Part model, mm, in its own coordinate system. Face numbers are marked on the shaded views. A direction names the side the tool comes from. Give positions to 0.01 mm unless a question says otherwise; leave off trailing zeros. Loops run counter-clockwise (first coordinate to the right, second up) from the corner with the lowest first, then second, coordinate; pieces in that order, holes last. Notation, with made-up numbers: M 65,61 L 97,61 A17 ccw 97,87 Z; hole C 14.25,-11.75 d9. An arc over 180 degrees is marked long. Answer in a Markdown table with one row per item.
from build123d import *

# Parameters (mm, degrees)
F1_DEPTH     = 21.2
F2_W         = 14.7
F2_H         = 3.2
F3_DEPTH     = 6.7
F4_R         = 2.6
F5_DEPTH     = 10
F6_W         = 18
F6_H         = 15
F7_DEPTH     = 11.9
F9_DEPTH     = 7.6
F10_T1_DEPTH = 34.5
F10_T3_DEPTH = 27
F11_W        = 14.7
F11_H        = 1.8
F12_DEPTH    = 3.5


# Not quite as in the source:
# - a fillet or chamfer that OpenCascade refuses, or shapes differently, is made with other operations: its cross-section is extruded or revolved along the edge and cut away or added


with BuildPart() as f1:
    # F0 (on Front) → F1 (new body)
    with BuildSketch(Plane.XZ):
        with BuildLine():
            Line((-7.35, 0.194197055), (-7.35, -7.15))
            Line((-7.35, -7.15), (7.35, -7.15))
            Line((7.35, -7.15), (7.35, 0.194197055))
            Line((7.35, 0.194197055), (6.2603328375, 2.1552506672))
            ThreePointArc((6.2603328375, 2.1552506672), (3.3980247264, -0.3840505852), (0, 1.375007837))
            ThreePointArc((0, 1.375007837), (-3.3980247264, -0.3840505852), (-6.2603328375, 2.1552506672))
            Line((-6.2603328375, 2.1552506672), (-7.35, 0.194197055))
        make_face()
        with BuildLine():
            ThreePointArc((0, 4.564992163), (-4.1941925187, 6.1243837001), (-6.2603328375, 2.1552506672))
            ThreePointArc((-6.2603328375, 2.1552506672), (-3.3980247264, -0.3840505852), (0, 1.375007837))
            ThreePointArc((0, 1.375007837), (3.3980247264, -0.3840505852), (6.2603328375, 2.1552506672))
            ThreePointArc((6.2603328375, 2.1552506672), (4.1941925187, 6.1243837001), (0, 4.564992163))
        make_face()
    extrude(amount=F1_DEPTH)

    # F2 (on face) → F3 (cut)
    with BuildSketch(Plane(origin=(0, 0, -7.15), x_dir=(1, 0, 0), z_dir=(0, 0, -1))):
        with Locations((0, 19.6)):
            Rectangle(F2_W, F2_H)
    extrude(amount=-F3_DEPTH, mode=Mode.SUBTRACT)

    # F4 (on face) → F5 (cut)
    with BuildSketch(Plane.XZ.offset(21.2)):
        with Locations((-2.98, 2.97)):
            Circle(F4_R)
        with Locations((2.98, 2.97)):
            Circle(F4_R)
    extrude(amount=-F5_DEPTH, mode=Mode.SUBTRACT)

    # F6 (on face) → F7 (join)
    with BuildSketch(Plane(origin=(0, 0, 0), x_dir=(-1, 0, 0), z_dir=(0, 1, 0))):
        with Locations((0, 3.95)):
            Rectangle(F6_W, F6_H)
    extrude(amount=F7_DEPTH)

    # F8 (on face) → F9 (join)
    with BuildSketch(Plane(origin=(0, 11.9, 0), x_dir=(-1, 0, 0), z_dir=(0, 1, 0))):
        Polygon((-9, -0.05), (-9, -3.55), (9, -3.55), (9, -0.05), (11, -0.05), (11, 7.95), (9, 7.95), (9, 11.45), (-9, 11.45), (-9, 7.95), (-11, 7.95), (-11, -0.05), align=None)
    extrude(amount=F9_DEPTH)

    # F10: fillet of radius 3 on 4 edges, made by hand

    # F10_s2 → F10_t1 (cut)
    with BuildSketch(Plane.XZ.offset(-27)):
        with BuildLine():
            ThreePointArc((6, 11.45), (8.1213203436, 10.5713203436), (9, 8.45))
            Line((9, 8.45), (9, 11.45))
            Line((9, 11.45), (6, 11.45))
        make_face()
        with BuildLine():
            ThreePointArc((-9, 8.45), (-8.1213203436, 10.5713203436), (-6, 11.45))
            Line((-6, 11.45), (-9, 11.45))
            Line((-9, 11.45), (-9, 8.45))
        make_face()
    extrude(amount=F10_T1_DEPTH, mode=Mode.SUBTRACT)

    # F10_s4 → F10_t3 (cut)
    with BuildSketch(Plane.XZ.offset(-27)):
        with BuildLine():
            ThreePointArc((6, -3.55), (8.1213203436, -2.6713203436), (9, -0.55))
            Line((9, -0.55), (9, -3.55))
            Line((9, -3.55), (6, -3.55))
        make_face()
        with BuildLine():
            ThreePointArc((-6, -3.55), (-8.1213203436, -2.6713203436), (-9, -0.55))
            Line((-9, -0.55), (-9, -3.55))
            Line((-9, -3.55), (-6, -3.55))
        make_face()
    extrude(amount=F10_T3_DEPTH, mode=Mode.SUBTRACT)

    # F11 (on face) → F12 (cut)
    with BuildSketch(Plane(origin=(0, 0, -7.15), x_dir=(1, 0, 0), z_dir=(0, 0, -1))):
        with Locations((0, 17.1)):
            Rectangle(F11_W, F11_H)
    extrude(amount=-F12_DEPTH, mode=Mode.SUBTRACT)


solid = f1.part
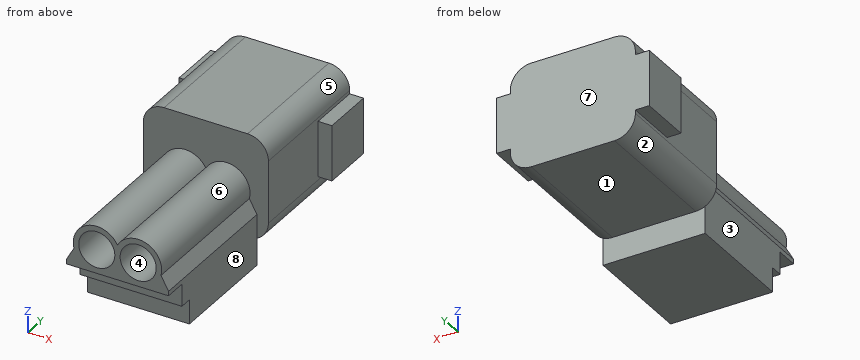
(1) Saw through at C-C (z = 3.75). Write the cut outline in (x, y).
Recorded:
| item | result |
|---|---|
| outline | M -11,11.9 L -9,11.9 L -9,0 L -6.27,0 L -6.27,-21.2 L -5.46,-21.2 L -5.46,-11.2 L -0.5,-11.2 L -0.5,-21.2 L 0.5,-21.2 L 0.5,-11.2 L 5.46,-11.2 L 5.46,-21.2 L 6.27,-21.2 L 6.27,0 L 9,0 L 9,11.9 L 11,11.9 L 11,19.5 L -11,19.5 Z |
(2) Saw through at A-A (x = 2.98). Write the cut outline in (y, z).
Recorded:
| item | result |
|---|---|
| outline | M -21.2,-0.45 L -18,-0.45 L -18,-3.65 L -16.2,-3.65 L -16.2,-7.15 L 0,-7.15 L 0,-3.55 L 19.5,-3.55 L 19.5,11.45 L 0,11.45 L 0,6.35 L -21.2,6.35 L -21.2,5.57 L -11.2,5.57 L -11.2,0.37 L -21.2,0.37 Z |
(3) Saw through at D-D (y = -12.5). Write the cut outline in (x, z) (3 decimals).
Recorded:
| item | result |
|---|---|
| outline | M -7.35,-7.15 L 7.35,-7.15 L 7.35,0.194 L 6.26,2.155 A3.38 ccw 0,4.565 A3.38 ccw -6.26,2.155 L -7.35,0.194 Z; hole C -2.98,2.97 d5.2; hole C 2.98,2.97 d5.2 |
(4) Pin check, flat tips, straight feed: pin 1 Ø2 at (y, z) = (-16, -4.5) entering from -X; pin 2 Ø1.4 at (x, y) = (3.5, -17) entering from -Z; pin 3 Ø3.5 at (y, z) = (-9, -3) entering from +X. Stop position of each tip, or through.
Recorded:
| item | result |
|---|---|
| pin 1 | stops at x = -7.35 |
| pin 2 | stops at z = -3.65 |
| pin 3 | stops at x = 7.35 |
(5) Which spindle directions (+Z, -Z, +X, -X, +Y, -Y) get a long thin tool onto all of the face, cutting with end or side? Do the marked faces 1, 2, 3, 4 and 5. Say none if no direction does.
Recorded:
| item | result |
|---|---|
| face 1 | -Z, +X, -X, +Y |
| face 2 | -Z, -X, +Y |
| face 3 | +Z, -Z, -X, -Y |
| face 4 | -Y |
| face 5 | +Z, +X, +Y, -Y |
(6) Drill centre lines: line 1 along Y through (x, z) = (6.25, -2.75); line 2 along Y through (x, z) = (-6.75, -4); line 3 along Z through (x, y) = (-2.98, -14.75). Where is each one in solid material? Low to high.
Recorded:
| item | result |
|---|---|
| line 1 | y = -18 to 19.5 |
| line 2 | y = -16.2 to 0 |
| line 3 | z = -7.15 to 0.37, 5.57 to 6.35 |
(7) Pull direction X, two halves, no side cores. Call the marked faces 6, 7 and 8: +X half, -X half, draft (parallel to the pull), parting line (faces both ways), or undercut.
Recorded:
| item | result |
|---|---|
| face 6 | undercut |
| face 7 | draft |
| face 8 | +X half |
(8) Saw through at B-B (y = 16). Write the cut outline in (x, z), plus the area to 3 significant figures.
Recorded:
| item | result |
|---|---|
| outline | M -11,-0.05 L -9,-0.05 L -9,-0.55 A3 ccw -6,-3.55 L 6,-3.55 A3 ccw 9,-0.55 L 9,-0.05 L 11,-0.05 L 11,7.95 L 9,7.95 L 9,8.45 A3 ccw 6,11.45 L -6,11.45 A3 ccw -9,8.45 L -9,7.95 L -11,7.95 Z |
| area | 294 mm^2 |
